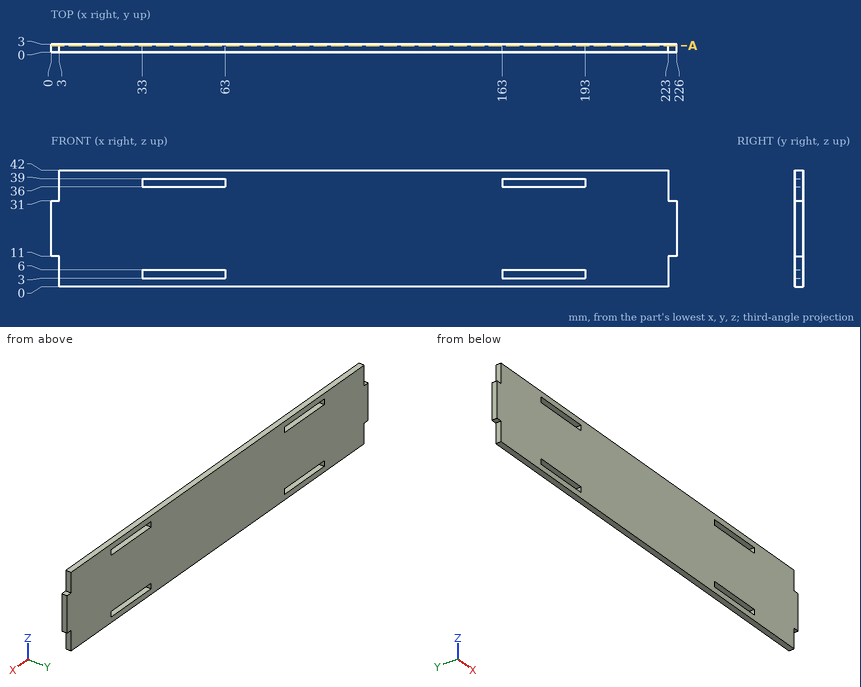
Print and shaded views of the part. All mm, measured from the part's lowest x, y and z. Coordinates: 2 decimals unless noted, no trailing zeros. Order: outer loops, then holes, each group sorted by start corner. A loop starts at its lowest first (then second) coordinate and runs counter-clockwise, first axis right, second up.
(1) Pin check, flat tips, straight feed: pin 1 Ø1.5 at (y, z) = (1, 38) entering from +X; pin 2 Ø1.5 at (x, y) = (2, 1.5) entering from +Z; pin 3 Ø1.5 at (y, z) = (1, 5.5) entering from -X. Stop position of each tip, or through.
Check sheet entries:
pin 1: stops at x = 223
pin 2: stops at z = 31
pin 3: stops at x = 3
(2) Slice it at A-A, the plane y = 2.45. Write the cut outline in (x, z).
Check sheet entries:
outline: (0, 11) - (3, 11) - (3, 0) - (223, 0) - (223, 11) - (226, 11) - (226, 31) - (223, 31) - (223, 42) - (3, 42) - (3, 31) - (0, 31) - close; hole (33, 3) - (63, 3) - (63, 6) - (33, 6) - close; hole (33, 36) - (63, 36) - (63, 39) - (33, 39) - close; hole (163, 3) - (193, 3) - (193, 6) - (163, 6) - close; hole (163, 36) - (193, 36) - (193, 39) - (163, 39) - close
(3) Probe L1, parallel to Z at x = 56, y = 2.65; L2, parallel to X at y = 0.55, z = 40. List the from-to ranges inside material, lowest first.
Check sheet entries:
L1: z = 0 to 3, 6 to 36, 39 to 42
L2: x = 3 to 223
